Autodesk Inventor part; units mm, degrees
ref_plane "YZ Plane" through (0, 0, 0) normal (1, 0, 0) x (0, 1, 0)
ref_plane "XZ Plane" through (0, 0, 0) normal (0, 1, 0) x (-1, 0, 0)
ref_plane "XY Plane" through (0, 0, 0) normal (0, 0, 1) x (1, 0, 0)
sketch "Sketch1" plane through (0, 0, 0) normal (0, 0, 1) x (1, 0, 0)
  arc A0 (0, 90) -> (77.9423, -45) centre (0, 0) ccw
  arc A1 (0, 25) -> (21.6506, -12.5) centre (0, 0) ccw
  line L0 (0, 25) -> (0, 90)
  line L1 (77.9423, -45) -> (21.6506, -12.5)
  line L2 (0, 25) -> (0, 0)
  line L3 (0, 0) -> (21.6506, -12.5)
  line L4 (0, -167.6192) -> (0, 145.1192)
  dimension "d0" = 120
  dimension "d1" = 25
  dimension "d2" = 90
extrude "Extrusion1" add sketch "Sketch1" along normal blind 4 contours L0 A1 L4 A0 | L4 A1 L1 A0
sketch "Sketch2" plane through (0, 0, 0) normal (0, 0, -1) x (-1, 0, 0)
  circle A0 centre (6.9725, 79.6956) radius 1.5
  circle A1 centre (20.7055, 77.2741) radius 1.5
  circle A2 centre (6.9459, 39.3923) radius 1.5
  line L0 (6.9725, 79.6956) -> (0, 0)
  line L1 (0, 0) -> (6.9459, 39.3923)
  line L2 (20.7055, 77.2741) -> (0, 0)
  line L3 (0, 25) -> (0, 90)
  dimension "d14" = 3
  dimension "d15" = 3
  dimension "d16" = 3
  dimension "d17" = 80
  dimension "d18" = 80
  dimension "d19" = 40
  dimension "d20" = 10
  dimension "d21" = 5
  dimension "d22" = 15
extrude "Extrusion2" cut sketch "Sketch2" against normal blind 10
pattern_circular "Circular Pattern1" count 12 over 220 about axis through (0, 0, 0) along (0, 0, 1) of "Extrusion2"
sketch "Sketch3" plane through (0, 0, 4) normal (0, 0, 1) x (1, 0, 0)
  point P0 (0, 0)
sketch "Sketch4" plane through (0, 0, 4) normal (0, 0, 1) x (1, 0, 0)
  arc A0 (0, 25) -> (21.6506, -12.5) centre (0, 0) ccw
  line L0 (0, 0) -> (-30.7818, 84.5723)
  line L1 (0, 25) -> (0, 90)
  line L2 (0, 0) -> (77.9423, -45)
  arc A1 (-30.7818, 84.5723) -> (77.9423, -45) centre (0, 0) ccw
  point P0 (21.6506, -12.5)
  point P1 (-8.5505, 23.4923)
  dimension "d29" = 20
extrude "Extrusion3" cut sketch "Sketch4" against normal blind 10 contours A0 L2 A1 L0
properties part number "cover"
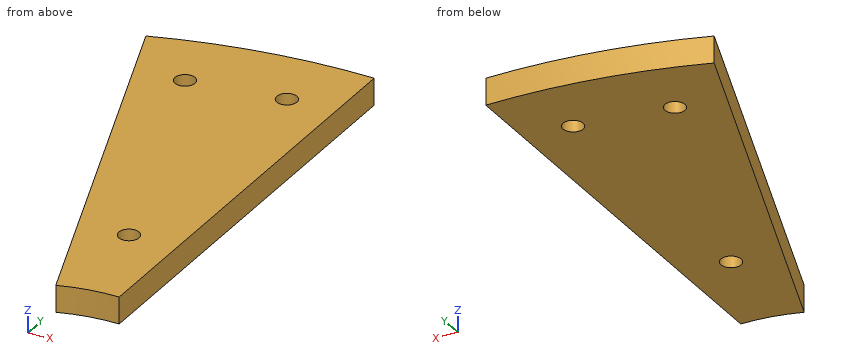
Check sheet for the modelled part. Datum: model origin and axes. Units: mm. Coordinates: 2 decimals unless noted, no trailing zeros. Loops run counter-clockwise (first coordinate to the right, second up) from the corner with the lowest first, then second, coordinate; pieces in that order, holes last. Notation, with made-up numbers: (17, 79) -> (64, 79) arc R13 cw to (64, 92) -> close; hole circle Ø7 at (-5, 32). An arc over 180 degrees is marked (long way). Write item = value, one per line. Start each with the question number.
1. Section check A-A on z = 3.15. Record the cut outline in (x, y).
2. Material ranges on line 1 (Y direction, x = -7, z = 1.4); line 2 (Y direction, x = -6, z = 2.8); line 3 (Y direction, x = -0.5, z = 1.5) (3 decimals), recorded low to high.
3. Section check B-B on y = 67.5. Record the cut outline in (x, z), then the cut area to 3 significant figures.
4. Section check C-C on x = -24. Record the cut outline in (y, z).
Responses:
q1.outline = (-30.78, 84.57) -> (-8.55, 23.49) arc R25 cw to (0, 25) -> (0, 90) arc R90 ccw to start; hole circle Ø3 at (-20.71, 77.27); hole circle Ø3 at (-6.97, 79.7); hole circle Ø3 at (-6.95, 39.39)
q2.line_1 = 24 to 37.89, 40.89 to 78.2, 81.2 to 89.73
q2.line_2 = 24.27 to 38.23, 40.56 to 78.55, 80.84 to 89.8
q2.line_3 = 24.995 to 89.999
q3.outline = (-24.57, 0) -> (0, 0) -> (0, 4) -> (-24.57, 4) -> close
q3.area = 98.3 mm2
q4.outline = (65.94, 0) -> (86.74, 0) -> (86.74, 4) -> (65.94, 4) -> close
